```python
from build123d import *

# Parameters (mm, degrees)
F0_R     = 2.75
F1_DEPTH = 4
F2_W     = 16.5
F2_H     = 16.5
F3_DEPTH = 4.5
F4_W     = 26.5
F4_H     = 22.7
F4_W_2   = 16.5
F4_H_2   = 12.7
F5_DEPTH = 2.5
F7_SIZE  = 0.5


with BuildPart() as f1:
    # F0 (on Front) → F1 (new body)
    with BuildSketch(Plane.XZ):
        with BuildLine():
            ThreePointArc((40, -6.35), (46.35, 0), (40, 6.35))
            Line((40, 6.35), (-40, 6.35))
            ThreePointArc((-40, 6.35), (-46.35, 0), (-40, -6.35))
            Line((-40, -6.35), (40, -6.35))
        make_face()
        with Locations((-40, 0)):
            Circle(F0_R, mode=Mode.SUBTRACT)
        with Locations((40, 0)):
            Circle(F0_R, mode=Mode.SUBTRACT)
    extrude(amount=-F1_DEPTH)

    # F2 (on Front) → F3 (join)
    with BuildSketch(Plane.XZ):
        Rectangle(F2_W, F2_H)
    extrude(amount=F3_DEPTH)

    # F4 (on face) → F5 (cut)
    with BuildSketch(Plane.XZ):
        Rectangle(F4_W, F4_H)
        Rectangle(F4_W_2, F4_H_2, mode=Mode.SUBTRACT)
    extrude(amount=F5_DEPTH, mode=Mode.SUBTRACT)

    # F7
    f7_edges = [f1.edges().sort_by_distance(p)[0] for p in [
        (8.25, -4.5, 0),
        (0, -4.5, 8.25),
        (-8.25, -4.5, 0),
        (0, -4.5, -8.25),
        (8.25, -3.5, 8.25),
        (-8.25, -3.5, 8.25),
        (-8.25, -3.5, -8.25),
        (8.25, -3.5, -8.25),
        (46.35, 4, 0),
        (0, 4, 6.35),
        (-46.35, 4, 0),
        (0, 4, -6.35),
        (-42.75, 4, 0),
        (37.25, 4, 0),
        (0, -2.5, 8.25),
        (8.25, -2.5, -7.3),
        (8.25, -2.5, 7.3),
        (-8.25, -2.5, 7.3),
        (-8.25, -2.5, -7.3),
        (0, -2.5, -8.25),
        (24.125, 0, 6.35),
        (37.25, 0, 0),
        (8.25, -1.25, 6.35),
        (8.25, -1.25, -6.35),
        (-8.25, -1.25, 6.35),
        (-8.25, -1.25, -6.35),
        (-24.125, 0, -6.35),
        (-42.75, 0, 0),
        (46.35, 0, 0),
        (-46.35, 0, 0),
        (-24.125, 0, 6.35),
        (24.125, 0, -6.35),
    ]]
    chamfer(f7_edges, length=F7_SIZE)


solid = f1.part
```
Geometry check sheet. Reference: the model listing, model coordinates, mm. A direction names the side the tool comes from. Coordinates: 2 decimals unless noted, no trailing zeros. Order: outer loops, then holes, each group sorted by start corner. A loop starts at its lowest first (then second) coordinate and runs counter-clockwise, first axis right, second up. Notation, with made-up numbers: (84.25, 21.5) - (89.25, 21.5) arc R24 cw to (89.25, 50.5) - close; hole circle Ø1 at (65, 26.5). An arc over 180 degrees is marked (long way). Answer as a JSON object with one key per item and string values. Group by question number.
Item 1: Depth check by flat-ended pin: pin 1 Ø4.5 at (y, z) = (-3, -3) entering from -X; pin 2 Ø3 at (x, y) = (19.5, 0.5) entering from +Z; pin 3 Ø4.5 at (y, z) = (-2, -3) entering from +X. Enter the tip coordinate at first touch or a pass-through.
Item 2: Sectioned sample at A-A, the plane z = 0. Give the number of separate pieces and of enclosed holes in the cut face, and give its area (3 significant figures).
Item 3: Tool access check on faces 4 (the face through (-1, 2, -6.35)), 5 (the face through (-1, 2, 6.35)), 6 (the face through (-27, 0, 0)), 7 (the face through (8.25, -2, 0)), 8 (the face through (46.35, 1.98, -0.14)). Record the directions out of +Z, -Z, +X, -X, +Y, -Y that give a thin tool (end or side, any length) a straight path to the whole face; none if there is none.
Item 4: Sectioned sample at B-B, the plane x = -5.5. Record the cut outline in (y, z), and give its area (3 significant figures).
Item 5: Sectioned sample at C-C, the plane x = 27. Record the cut outline in (y, z), and give its area (3 significant figures).
Item 6: Scan lines: probe 1 along Z at (x, y) = (40, 1.9); probe 2 along X at (y, z) = (1, 0.75); probe 3 along Z at (x, y) = (-29, 1). Record each from-to range of solid material in increasing order.
Item 7: Draft check along Z on faces 1 (the face through (-45.99, 3.86, 0.13)), 2 (the face through (37.253, 1.979, 0.121)), 3 (the face through (-8.25, -2, 0)). Enter one of: +Z half, -Z half, draft (parallel to the pull), parting line (faces both ways), or undercut.
Resolved:
{
 "1": {"pin 1": "x = -8.25", "pin 2": "z = 6.35", "pin 3": "x = 45.53"},
 "2": {"separate pieces": "3", "enclosed holes": "0", "area": "399 mm^2"},
 "3": {"face 4": "-Z, +X, -X, +Y", "face 5": "+Z, +X, -X, +Y", "face 6": "+Z, -Z, -X, -Y", "face 7": "+Z, -Z, +X, -Y", "face 8": "+X, +Y, -Y"},
 "4": {"outline": "(-4.5, -7.75) - (-4, -8.25) - (-3, -8.25) - (-2.5, -7.75) - (-2.5, -6.35) - (3.5, -6.35) - (4, -5.85) - (4, 5.85) - (3.5, 6.35) - (-2.5, 6.35) - (-2.5, 7.75) - (-3, 8.25) - (-4, 8.25) - (-4.5, 7.75) - close", "area": "115 mm^2"},
 "5": {"outline": "(0, -5.85) - (0.5, -6.35) - (3.5, -6.35) - (4, -5.85) - (4, 5.85) - (3.5, 6.35) - (0.5, 6.35) - (0, 5.85) - close", "area": "50.3 mm^2"},
 "6": {"probe 1": "-6.35 to -2.75, 2.75 to 6.35", "probe 2": "-46.31 to -42.65, -37.35 to 37.35, 42.65 to 46.31", "probe 3": "-6.35 to 6.35"},
 "7": {"face 1": "parting line", "face 2": "undercut", "face 3": "draft"}
}
